Source: CAD feature listing. Evaluate the final solid. Frame: model axes, mm. A direction names the side the tool comes from. Give positions to 0.01 mm unless a question says otherwise; leave off trailing zeros. Write each loop counter-clockwise with the first axis right and the second up, starting at its lowest first coordinate (ties: lowest second). Pieces come first, ordered by that corner, then holes.
```python
from build123d import *

# Parameters (mm, degrees)
SKIZZE1_W                            = 25
SKIZZE1_H                            = 75
AUFSATZ_LINEAR_AUSTRAGEN1_DEPTH      = 4.8
SCHNITT_LINEAR_AUSTRAGEN1_DEPTH      = 5
SKIZZE3_W                            = 25
SKIZZE3_H                            = 25
SCHNITT_LINEAR_AUSTRAGEN2_DEPTH      = 1
SKIZZE4_W                            = 15
SKIZZE4_H                            = 23
SCHNITT_LINEAR_AUSTRAGEN3_DEPTH      = 2
SKIZZE5_R                            = 4
SCHNITT_LINEAR_AUSTRAGEN4_DEPTH      = 2.8
SKIZZE6_W                            = 10
SKIZZE6_H                            = 10
SKIZZE6_R                            = 4
SCHNITT_LINEAR_AUSTRAGEN5_DEPTH      = 1.5
AUFSATZ_LINEAR_AUSTRAGEN2_DEPTH      = 6
SKIZZE8_R                            = 2
SCHNITT_LINEAR_AUSTRAGEN6_DEPTH      = 2.2
SCHNITT_LINEAR_AUSTRAGEN6_DEPTH_BACK = 5.8
SKIZZE9_W                            = 6.6
SKIZZE9_H                            = 19
SCHNITT_LINEAR_AUSTRAGEN7_DEPTH      = 5.8
AUFSATZ_LINEAR_AUSTRAGEN3_DEPTH      = 4.8
VERRUNDUNG1_R                        = 2
VERRUNDUNG2_R                        = 1
SCHNITT_LINEAR_AUSTRAGEN8_DEPTH      = 5.8000001
VERRUNDUNG3_R                        = 1


with BuildPart() as part:
    # Skizze1 → Aufsatz-Linear austragen1 (new body)
    with BuildSketch(Plane.XY):
        with Locations((0, 37.5)):
            Rectangle(SKIZZE1_W, SKIZZE1_H)
    extrude(amount=AUFSATZ_LINEAR_AUSTRAGEN1_DEPTH)

    # Skizze2 → Schnitt-Linear austragen1 (cut)
    with BuildSketch(Plane.XY.offset(4.8)):
        with BuildLine():
            ThreePointArc((-9.4, 73), (-11.277817459, 73.777817459), (-10.5, 71.9))
            Line((-10.5, 71.9), (-10.5, 73))
            Line((-10.5, 73), (-9.4, 73))
        make_face()
        with BuildLine():
            Line((-10.5, 73), (-10.5, 71.9))
            ThreePointArc((-10.5, 71.9), (-9.722182541, 72.222182541), (-9.4, 73))
            Line((-9.4, 73), (-10.5, 73))
        make_face()
        with BuildLine():
            ThreePointArc((9.4, 73), (9.722182541, 72.222182541), (10.5, 71.9))
            Line((10.5, 71.9), (10.5, 73))
            Line((10.5, 73), (9.4, 73))
        make_face()
        with BuildLine():
            Line((10.5, 73), (10.5, 71.9))
            ThreePointArc((10.5, 71.9), (11.277817459, 72.222182541), (11.6, 73))
            ThreePointArc((11.6, 73), (10.5, 74.1), (9.4, 73))
            Line((9.4, 73), (10.5, 73))
        make_face()
        with BuildLine():
            ThreePointArc((9.4, 73), (9.722182541, 72.222182541), (10.5, 71.9))
            Line((10.5, 71.9), (10.5, 73))
            Line((10.5, 73), (9.4, 73))
        make_face()
        with BuildLine():
            Line((10.5, 73), (10.5, 71.9))
            ThreePointArc((10.5, 71.9), (11.277817459, 72.222182541), (11.6, 73))
            ThreePointArc((11.6, 73), (10.5, 74.1), (9.4, 73))
            Line((9.4, 73), (10.5, 73))
        make_face()
        with BuildLine():
            ThreePointArc((-10.5, 61.6), (-11.277817459, 59.722182541), (-9.4, 60.5))
            Line((-9.4, 60.5), (-10.5, 60.5))
            Line((-10.5, 60.5), (-10.5, 61.6))
        make_face()
        with BuildLine():
            Line((-10.5, 60.5), (-9.4, 60.5))
            ThreePointArc((-9.4, 60.5), (-9.722182541, 61.277817459), (-10.5, 61.6))
            Line((-10.5, 61.6), (-10.5, 60.5))
        make_face()
        with BuildLine():
            ThreePointArc((-10.5, 61.6), (-11.277817459, 59.722182541), (-9.4, 60.5))
            Line((-9.4, 60.5), (-10.5, 60.5))
            Line((-10.5, 60.5), (-10.5, 61.6))
        make_face()
        with BuildLine():
            Line((-10.5, 60.5), (-9.4, 60.5))
            ThreePointArc((-9.4, 60.5), (-9.722182541, 61.277817459), (-10.5, 61.6))
            Line((-10.5, 61.6), (-10.5, 60.5))
        make_face()
        with BuildLine():
            ThreePointArc((10.5, 61.6), (9.722182541, 61.277817459), (9.4, 60.5))
            Line((9.4, 60.5), (10.5, 60.5))
            Line((10.5, 60.5), (10.5, 61.6))
        make_face()
        with BuildLine():
            Line((10.5, 60.5), (9.4, 60.5))
            ThreePointArc((9.4, 60.5), (10.5, 59.4), (11.6, 60.5))
            ThreePointArc((11.6, 60.5), (11.277817459, 61.277817459), (10.5, 61.6))
            Line((10.5, 61.6), (10.5, 60.5))
        make_face()
        with BuildLine():
            ThreePointArc((10.5, 61.6), (9.722182541, 61.277817459), (9.4, 60.5))
            Line((9.4, 60.5), (10.5, 60.5))
            Line((10.5, 60.5), (10.5, 61.6))
        make_face()
        with BuildLine():
            Line((10.5, 60.5), (9.4, 60.5))
            ThreePointArc((9.4, 60.5), (10.5, 59.4), (11.6, 60.5))
            ThreePointArc((11.6, 60.5), (11.277817459, 61.277817459), (10.5, 61.6))
            Line((10.5, 61.6), (10.5, 60.5))
        make_face()
        with BuildLine():
            ThreePointArc((-9.4, 73), (-11.277817459, 73.777817459), (-10.5, 71.9))
            Line((-10.5, 71.9), (-10.5, 73))
            Line((-10.5, 73), (-9.4, 73))
        make_face()
        with BuildLine():
            Line((-10.5, 73), (-10.5, 71.9))
            ThreePointArc((-10.5, 71.9), (-9.722182541, 72.222182541), (-9.4, 73))
            Line((-9.4, 73), (-10.5, 73))
        make_face()
    extrude(amount=-SCHNITT_LINEAR_AUSTRAGEN1_DEPTH, mode=Mode.SUBTRACT)

    # Skizze3 → Schnitt-Linear austragen2 (cut)
    with BuildSketch(Plane.XY.offset(4.8)):
        with Locations((0, 62.5)):
            Rectangle(SKIZZE3_W, SKIZZE3_H)
    extrude(amount=-SCHNITT_LINEAR_AUSTRAGEN2_DEPTH, mode=Mode.SUBTRACT)

    # Skizze4 → Schnitt-Linear austragen3 (cut)
    with BuildSketch(Plane.XY.offset(3.8)):
        with Locations((0, 61.5)):
            Rectangle(SKIZZE4_W, SKIZZE4_H)
    extrude(amount=-SCHNITT_LINEAR_AUSTRAGEN3_DEPTH, mode=Mode.SUBTRACT)

    # Skizze5 → Schnitt-Linear austragen4 (cut, through all)
    with BuildSketch(Plane.XY.offset(1.8)):
        with Locations((0, 60.6)):
            Circle(SKIZZE5_R)
    extrude(amount=-SCHNITT_LINEAR_AUSTRAGEN4_DEPTH, mode=Mode.SUBTRACT)

    # Skizze6 → Schnitt-Linear austragen5 (cut)
    with BuildSketch(Plane.XY.offset(1.8)):
        with Locations((0, 60.6)):
            Rectangle(SKIZZE6_W, SKIZZE6_H)
        with Locations((0, 60.6)):
            Circle(SKIZZE6_R, mode=Mode.SUBTRACT)
    extrude(amount=-SCHNITT_LINEAR_AUSTRAGEN5_DEPTH, mode=Mode.SUBTRACT)

    # Skizze7 → Aufsatz-Linear austragen2 (add)
    with BuildSketch(Plane.XY):
        with BuildLine():
            ThreePointArc((-10.5, 61.6), (-11.277817459, 59.722182541), (-9.4, 60.5))
            Line((-9.4, 60.5), (-10.5, 60.5))
            Line((-10.5, 60.5), (-10.5, 61.6))
        make_face()
        with BuildLine():
            Line((-10.5, 60.5), (-9.4, 60.5))
            ThreePointArc((-9.4, 60.5), (-9.722182541, 61.277817459), (-10.5, 61.6))
            Line((-10.5, 61.6), (-10.5, 60.5))
        make_face()
        with BuildLine():
            ThreePointArc((-9.4, 73), (-11.277817459, 73.777817459), (-10.5, 71.9))
            Line((-10.5, 71.9), (-10.5, 73))
            Line((-10.5, 73), (-9.4, 73))
        make_face()
        with BuildLine():
            Line((-10.5, 73), (-10.5, 71.9))
            ThreePointArc((-10.5, 71.9), (-9.722182541, 72.222182541), (-9.4, 73))
            Line((-9.4, 73), (-10.5, 73))
        make_face()
        with BuildLine():
            ThreePointArc((10.5, 61.6), (9.722182541, 61.277817459), (9.4, 60.5))
            Line((9.4, 60.5), (10.5, 60.5))
            Line((10.5, 60.5), (10.5, 61.6))
        make_face()
        with BuildLine():
            Line((10.5, 60.5), (9.4, 60.5))
            ThreePointArc((9.4, 60.5), (10.5, 59.4), (11.6, 60.5))
            ThreePointArc((11.6, 60.5), (11.277817459, 61.277817459), (10.5, 61.6))
            Line((10.5, 61.6), (10.5, 60.5))
        make_face()
        with BuildLine():
            ThreePointArc((9.4, 73), (9.722182541, 72.222182541), (10.5, 71.9))
            Line((10.5, 71.9), (10.5, 73))
            Line((10.5, 73), (9.4, 73))
        make_face()
        with BuildLine():
            Line((10.5, 73), (10.5, 71.9))
            ThreePointArc((10.5, 71.9), (11.277817459, 72.222182541), (11.6, 73))
            ThreePointArc((11.6, 73), (10.5, 74.1), (9.4, 73))
            Line((9.4, 73), (10.5, 73))
        make_face()
        with BuildLine():
            ThreePointArc((9.4, 73), (9.722182541, 72.222182541), (10.5, 71.9))
            Line((10.5, 71.9), (10.5, 73))
            Line((10.5, 73), (9.4, 73))
        make_face()
        with BuildLine():
            Line((10.5, 73), (10.5, 71.9))
            ThreePointArc((10.5, 71.9), (11.277817459, 72.222182541), (11.6, 73))
            ThreePointArc((11.6, 73), (10.5, 74.1), (9.4, 73))
            Line((9.4, 73), (10.5, 73))
        make_face()
        with BuildLine():
            ThreePointArc((10.5, 61.6), (9.722182541, 61.277817459), (9.4, 60.5))
            Line((9.4, 60.5), (10.5, 60.5))
            Line((10.5, 60.5), (10.5, 61.6))
        make_face()
        with BuildLine():
            Line((10.5, 60.5), (9.4, 60.5))
            ThreePointArc((9.4, 60.5), (10.5, 59.4), (11.6, 60.5))
            ThreePointArc((11.6, 60.5), (11.277817459, 61.277817459), (10.5, 61.6))
            Line((10.5, 61.6), (10.5, 60.5))
        make_face()
        with BuildLine():
            ThreePointArc((-10.5, 61.6), (-11.277817459, 59.722182541), (-9.4, 60.5))
            Line((-9.4, 60.5), (-10.5, 60.5))
            Line((-10.5, 60.5), (-10.5, 61.6))
        make_face()
        with BuildLine():
            Line((-10.5, 60.5), (-9.4, 60.5))
            ThreePointArc((-9.4, 60.5), (-9.722182541, 61.277817459), (-10.5, 61.6))
            Line((-10.5, 61.6), (-10.5, 60.5))
        make_face()
        with BuildLine():
            ThreePointArc((-9.4, 73), (-11.277817459, 73.777817459), (-10.5, 71.9))
            Line((-10.5, 71.9), (-10.5, 73))
            Line((-10.5, 73), (-9.4, 73))
        make_face()
        with BuildLine():
            Line((-10.5, 73), (-10.5, 71.9))
            ThreePointArc((-10.5, 71.9), (-9.722182541, 72.222182541), (-9.4, 73))
            Line((-9.4, 73), (-10.5, 73))
        make_face()
    extrude(amount=AUFSATZ_LINEAR_AUSTRAGEN2_DEPTH)

    # Skizze8 → Schnitt-Linear austragen6 (cut, two sides)
    with BuildSketch(Plane.XY.offset(4.8)) as schnitt_linear_austragen6_sk:
        with Locations((0, 5.5)):
            Circle(SKIZZE8_R)
    extrude(amount=SCHNITT_LINEAR_AUSTRAGEN6_DEPTH, mode=Mode.SUBTRACT)
    extrude(schnitt_linear_austragen6_sk.sketch, amount=-SCHNITT_LINEAR_AUSTRAGEN6_DEPTH_BACK, mode=Mode.SUBTRACT)

    # Skizze9 → Schnitt-Linear austragen7 (cut, through all)
    with BuildSketch(Plane.XY.offset(4.8)):
        with Locations((-9.2, 9.5)):
            Rectangle(SKIZZE9_W, SKIZZE9_H)
        with Locations((9.2, 9.5)):
            Rectangle(SKIZZE9_W, SKIZZE9_H)
    extrude(amount=-SCHNITT_LINEAR_AUSTRAGEN7_DEPTH, mode=Mode.SUBTRACT)

    # Skizze10 → Aufsatz-Linear austragen3 (add)
    with BuildSketch(Plane.XY.offset(4.8)):
        with BuildLine():
            ThreePointArc((-20.231626451, 11.490217952), (-13.594656371, 16.254350305), (-5.9, 19))
            Line((-5.9, 19), (-12.5, 19))
            Line((-12.5, 19), (-12.5, 29.567918994))
            ThreePointArc((-12.5, 29.567918994), (-14.514033208, 19.73708329), (-20.231626451, 11.490217952))
        make_face()
        with BuildLine():
            ThreePointArc((5.9, 19), (13.594656371, 16.254350305), (20.231626451, 11.490217952))
            ThreePointArc((20.231626451, 11.490217952), (14.514033208, 19.73708329), (12.5, 29.567918994))
            Line((12.5, 29.567918994), (12.5, 19))
            Line((12.5, 19), (5.9, 19))
        make_face()
    extrude(amount=-AUFSATZ_LINEAR_AUSTRAGEN3_DEPTH)

    # Verrundung1
    verrundung1_edges = [part.edges().sort_by_distance(p)[0] for p in [
        (-12.5, 75, 1.9),
        (12.5, 75, 1.9),
    ]]
    fillet(verrundung1_edges, radius=VERRUNDUNG1_R)

    # Verrundung2
    verrundung2_edges = [part.edges().sort_by_distance(p)[0] for p in [
        (-20.231626451, 11.490217952, 2.4),
        (20.231626451, 11.490217952, 2.4),
    ]]
    fillet(verrundung2_edges, radius=VERRUNDUNG2_R)

    # Skizze12 → Schnitt-Linear austragen8 (cut, through all)
    with BuildSketch(Plane.XY.offset(4.8)):
        Polygon((-1.884038216, 34.5), (-9.5, 44.521002347), (-9.5, 24.478997653), align=None)
        Polygon((0, 36.978997653), (7.615961784, 47), (-7.615961784, 47), align=None)
        Polygon((9.5, 24.478997653), (9.5, 44.521002347), (1.884038216, 34.5), align=None)
        with BuildLine():
            ThreePointArc((7.615961784, 22), (0, 22.902325259), (-7.615961784, 22))
            Line((-7.615961784, 22), (0, 32.021002347))
            Line((0, 32.021002347), (7.615961784, 22))
        make_face()
    extrude(amount=-SCHNITT_LINEAR_AUSTRAGEN8_DEPTH, mode=Mode.SUBTRACT)

    # Verrundung3
    verrundung3_edges = [part.edges().sort_by_distance(p)[0] for p in [
        (1.884038216, 34.5, 2.4),
        (9.5, 44.521002347, 2.4),
        (9.5, 24.478997653, 2.4),
        (0, 36.978997653, 2.4),
        (-7.615961784, 47, 2.4),
        (7.615961784, 47, 2.4),
        (7.615961784, 22, 2.4),
        (-7.615961784, 22, 2.4),
        (0, 32.021002347, 2.4),
        (-1.884038216, 34.5, 2.4),
        (-9.5, 24.478997653, 2.4),
        (-9.5, 44.521002347, 2.4),
    ]]
    fillet(verrundung3_edges, radius=VERRUNDUNG3_R)


solid = part.part
```
1. Cut plane A-A, the plane y = 5.5. Return the cut outline in (x, z).
2. Line query: L1, parallel to X at y = 71.5, z = 3; L2, parallel to Y at x = -5, z = 4.5; L3, parallel to X at y = 58.5, z = 1.5. Output: solid intervals per line, ascending.
3. Access query for faces 1 (the flat face through (5.9, 9, 2)), 2 (the flat face through (7.5, 61, 3)), 3 (the cylindrical face through (6.503, 46.43, 2.366)). Directions: +Z, -Z, +X, -X, +Y, -Y. A direction counts if a zero-diameter tool reaches every point of the face in a straight line with its end or side. Return the directions, or none.
4. Cut plane C-C, the plane y = 52.5. Return the cut outline in (x, z).
5. Cut plane D-D, the plane y = 32.5. Return the cut outline in (x, z).
6. Contact query for flat-ended pins moving along their axis: P1, Ø4, axis at x = -8.5, y = 39, coming from the +Z side; P2, Ø1, axis at y = 47, z = 2.5, coming from the -X side; P3, Ø7, axis at x = 0, y = 60.6, coming from the -Z side; P4, Ø1, axis at y = 26.5, z = 4.5, coming from the +X side. Output: stop coordinate, or through.
7. Mould query, pull axis Y, two halves, no side actions, for faces 4 (the flat face through (12.5, 51, 2)), 5 (the cylindrical face through (-11.93, 74.4, 1.93)), 6 (the flat face through (-3.445, 27.488, 2.434)). Classes: +Y half, -Y half, draft (parallel to the pull), parting line (faces both ways), or undercut.
8. Cut plane B-B, the plane x = 0. Return the cut outline in (y, z).
Response values:
1. outline: (-5.9, 0) - (-2, 0) - (-2, 4.8) - (-5.9, 4.8) - close; (2, 0) - (5.9, 0) - (5.9, 4.8) - (2, 4.8) - close
2. L1: x = -12.5 to -7.5, 7.5 to 12.5
2. L2: y = 0 to 22.52, 25.44 to 30.4, 38.6 to 43.56, 47 to 50
2. L3: x = -12.5 to -5, 5 to 12.5
3. face 1: +Z, -Z, -Y
3. face 2: +Z
3. face 3: +Z, -Z
4. outline: (-12.5, 0) - (12.5, 0) - (12.5, 3.8) - (7.5, 3.8) - (7.5, 1.8) - (-7.5, 1.8) - (-7.5, 3.8) - (-12.5, 3.8) - close
5. outline: (-12.5, 0) - (-9.5, 0) - (-9.5, 4.8) - (-12.5, 4.8) - close; (-3.4, 0) - (3.4, 0) - (3.4, 4.8) - (-3.4, 4.8) - close; (9.5, 0) - (12.5, 0) - (12.5, 4.8) - (9.5, 4.8) - close
6. P1: stops at z = 4.8
6. P2: stops at x = -12.5
6. P3: passes through
6. P4: stops at x = 12.76
7. face 4: draft
7. face 5: +Y half
7. face 6: undercut
8. outline: (0, 0) - (3.5, 0) - (3.5, 4.8) - (0, 4.8) - close; (7.5, 0) - (22.9, 0) - (22.9, 4.8) - (7.5, 4.8) - close; (31.37, 0) - (37.63, 0) - (37.63, 4.8) - (31.37, 4.8) - close; (47, 0) - (56.6, 0) - (56.6, 0.3) - (55.6, 0.3) - (55.6, 1.8) - (50, 1.8) - (50, 4.8) - (47, 4.8) - close; (64.6, 0) - (75, 0) - (75, 3.8) - (73, 3.8) - (73, 1.8) - (65.6, 1.8) - (65.6, 0.3) - (64.6, 0.3) - close
